Geometry check sheet. Reference: the model listing, model coordinates, mm. A direction names the side the tool comes from. Give positions to 0.01 mm unless a question says otherwise; leave off trailing zeros. Order: outer loops, then holes, each group sorted by start corner. A loop starts at its lowest first (then second) coordinate and runs counter-clockwise, first axis right, second up.
from build123d import *

# Parameters (mm, degrees)
BOSS_EXTRUDE1_DEPTH = 30
SKETCH2_R           = 15
BOSS_EXTRUDE2_DEPTH = 55
FILLET1_R           = 3.5
FILLET5_R           = 15
BOSS_EXTRUDE3_DEPTH = 20
SKETCH6_R           = 15
BOSS_EXTRUDE4_DEPTH = 40


with BuildPart() as part:
    # Sketch1 → Boss-Extrude1 (new body)
    with BuildSketch(Plane.XY):
        with BuildLine():
            Line((0, 0), (4.730174559, 0))
            Line((4.730174559, 0), (4.730174559, -30))
            Line((4.730174559, -30), (0, -30))
            ThreePointArc((0, -30), (-25.69148146, 20), (0, 70))
            Line((0, 70), (0, 50))
            ThreePointArc((0, 50), (-10.355339059, 25), (0, 0))
        make_face()
    extrude(amount=BOSS_EXTRUDE1_DEPTH)

    # Sketch2 → Boss-Extrude2 (add)
    with BuildSketch(Plane(origin=(4.730174559, 0, 0), x_dir=(0, 0, -1), z_dir=(1, 0, 0))):
        with Locations(Location((-15, -15, 0), (0, 0, 90))):
            Circle(SKETCH2_R)
    extrude(amount=BOSS_EXTRUDE2_DEPTH)

    # Fillet1
    fillet1_edges = [part.edges().sort_by_distance(p)[0] for p in [
        (2.36508728, 0, 30),
        (2.36508728, 0, 0),
    ]]
    fillet(fillet1_edges, radius=FILLET1_R)

    # Fillet5
    fillet5_edges = [part.edges().sort_by_distance(p)[0] for p in [
        (2.36508728, -30, 0),
        (2.36508728, -30, 30),
    ]]
    fillet(fillet5_edges, radius=FILLET5_R - 0.0001)  # a hair under: the kernel refuses the full size

    # Sketch5 → Boss-Extrude3 (add)
    with BuildSketch(Plane(origin=(0, 70, 0), x_dir=(0, 0, -1), z_dir=(0, 1, 0))):
        with BuildLine():
            Line((-30, 0), (-40, -48.989794856))
            Line((-40, -48.989794856), (-40, -63.989794856))
            ThreePointArc((-40, -63.989794856), (-15, -88.989794856), (10, -63.989794856))
            Line((10, -63.989794856), (10, -48.989794856))
            Line((10, -48.989794856), (0, 0))
            Line((0, 0), (-30, 0))
        make_face()
    extrude(amount=-BOSS_EXTRUDE3_DEPTH)

    # Sketch6 → Boss-Extrude4 (add)
    with BuildSketch(Plane(origin=(0, 70, 0), x_dir=(1, 0, 0), z_dir=(0, 1, 0))):
        with Locations(Location((63.989794856, -15, 0), (0, 0, 90))):
            Circle(SKETCH6_R)
    extrude(amount=BOSS_EXTRUDE4_DEPTH)


solid = part.part
Item 1: Gauge pin test, flat ends, axial feed: pin 1 (2 mm diameter, centred on y = 84, z = 1.5, fed in from -X); pin 2 (3 mm diameter, centred on x = 27.5, z = 19, fed in from +Y); pin 3 (24 mm diameter, centred on y = -8.5, z = 18.5, fed in from +X). Record the tip position at first contact, or that the pin passes through.
Reported:
pin 1: stops at x = 55.7
pin 2: stops at y = 70
pin 3: stops at x = 59.73
Item 2: Scan lines: L1, parallel to Y at x = 45, z = 23; L2, parallel to Y at x = 1.5, z = 22.5; L3, parallel to Y at x = 81.5, z = 1. Record each from-to range of solid material in increasing order.
Reported:
L1: y = -27.69 to -2.31, 50 to 70
L2: y = -27.99 to 0, 50 to 70
L3: y = 50 to 70
Item 3: Set-up check for faces 1 (the flat face through (24.84, 60.14, -5.07)), 2 (the flat face through (44, 50, 15)), 3 (the flat face through (4.73, -4, 27)), 4 (the flat face through (4.73, -4, 4)), 5 (the flat face through (59.73, -15, 15)): record each of +Z, -Z, +X, -X, +Y, -Y from which the full face is reachable in a straight line by a thin tool's end or side.
Reported:
face 1: -Z, -X, +Y, -Y
face 2: +Z, -Z, +X
face 3: +Z, +X
face 4: -Z, +X
face 5: +Z, -Z, +X, -Y
Item 4: Sectioned sample at B-B (y = 94). Enter the section's corners in (x, z).
Reported:
outline: circle Ø30 at (63.99, 15)
Item 5: Sectioned sample at C-C (x = 73.5). Enter the section's corners in (y, z), and give its area (3 significant figures).
Reported:
outline: (50, -8.12) - (70, -8.12) - (70, 3.4) - (110, 3.4) - (110, 26.6) - (70, 26.6) - (70, 38.12) - (50, 38.12) - close
area: 1,850 mm2
Item 6: Sectioned sample at A-A (x = 37.5). Enter the section's corners in (y, z).
Reported:
outline: circle Ø30 at (-15, 15); (50, -7.65) - (70, -7.65) - (70, 37.65) - (50, 37.65) - close
